Read the model definition and answer for the solid it produces. Units are mm, in the model's axes. A direction names the side the tool comes from. Give positions to 0.01 mm unless a question says otherwise; leave off trailing zeros. Order: outer loops, then holes, each group sorted by start corner. A loop starts at its lowest first (then second) coordinate and runs counter-clockwise, first axis right, second up. Notation, with made-up numbers: M -7.75,29 L 13.25,29 A10 ccw 13.25,43 Z; hole C 72,33.25 d6. An arc over 180 degrees is marked long. One line per item, written item: value. Start each with the question number.
from build123d import *

# Parameters (mm, degrees)
SKETCH1_R           = 1
BOSS_EXTRUDE1_DEPTH = 1.5
FILLET1_R           = 1
FILLET2_R           = 1
FILLET3_R           = 1


with BuildPart() as part:
    # Sketch1 → Boss-Extrude1 (new body)
    with BuildSketch(Plane.XY):
        with BuildLine():
            Line((13.648087548, 15.547724074), (13.648087548, 16.047724074))
            Line((13.648087548, 16.047724074), (-11.216055041, 18.650494389))
            ThreePointArc((-11.216055041, 18.650494389), (-12.440799912, 18.231633219), (-13.152546714, 17.150494389))
            Line((-13.152546714, 17.150494389), (-15.098105849, 17.150494389))
            Line((-15.098105849, 17.150494389), (-15.098105849, 16.150494389))
            Line((-15.098105849, 16.150494389), (-13.152546714, 16.150494389))
            ThreePointArc((-13.152546714, 16.150494389), (-11.545884817, 14.677878786), (-9.547553428, 15.547724074))
            Line((-9.547553428, 15.547724074), (13.648087548, 15.547724074))
        make_face()
        with Locations((-11.216055041, 16.650494389)):
            Circle(SKETCH1_R, mode=Mode.SUBTRACT)
    extrude(amount=BOSS_EXTRUDE1_DEPTH)

    # Fillet1
    fillet1_edges = [part.edges().sort_by_distance(p)[0] for p in [
        (-13.152546714, 16.150494389, 0.75),
    ]]
    fillet(fillet1_edges, radius=FILLET1_R)

    # Fillet2
    fillet2_edges = [part.edges().sort_by_distance(p)[0] for p in [
        (-13.152546714, 17.150494389, 0.75),
    ]]
    fillet(fillet2_edges, radius=FILLET2_R)

    # Fillet3
    fillet3_edges = [part.edges().sort_by_distance(p)[0] for p in [
        (-9.547553428, 15.547724074, 0.75),
    ]]
    fillet(fillet3_edges, radius=FILLET3_R)


solid = part.part
Q1. Find section C-C, the plane y = 18.35. Give the vertices of the cut face in (x, z), then the cut area to 3 significant figures.
Q2. Each of these flat-tipped pins is pushed along its axis until it touches: pin 1 (0.6 mm diameter, centred on x = -14.5, z = 0.5, fed in from +Y); pin 2 (0.8 mm diameter, centred on x = -2, z = 0.5, fed in from -Y). Where does it stop, or does it pass through?
Q3. Consider probe 1 along Y at (x, z) = (-10.75, 0.7); probe 2 along Y at (x, z) = (3.75, 0.7); probe 3 along Y at (x, z) = (-1, 0.3). Determine where each line is inside the solid, lowest interval first.
Q4. Determine the mould class of faces 1 (the cylindrical face through (-13.32, 17.28, 0.76)), 2 (the cylindrical face through (-11.49, 14.67, 0.74)), 3 (the cylindrical face through (-11.35, 17.64, 0.74)) for opening direction Y: released by +Y, released by -Y, zero draft, split by the parting line, or undercut.
Q5. A tool of negligible diameter and unlimited length cuts with its end or side. For faces 4 (the flat face through (-4, 17, 0)), 5 (the flat face through (2, 15.548, 1)), 6 (the flat face through (-14, 17.15, 1)), 7 (the flat face through (-4, 17, 1.5)), 8 (the flat face through (-14, 16.15, 1)), from which of +Z, -Z, +X, -X, +Y, -Y can it reach the whole face along a straight path? Write none if from no direction.
Q6. Find section A-A, the plane z = 0.8. Give the vertices of the cut face in (x, y), then the cut area to 3 significant figures.
Q7. Find section B-B, the plane x = 4.75. Give the vertices of the cut face in (y, z), then the cut area to 3 significant figures.
Evaluation:
1. outline: M -12.27,0 L -8.35,0 L -8.35,1.5 L -12.27,1.5 Z
1. area: 5.89 mm2
2. pin 1: y = 17.15
2. pin 2: y = 15.55
3. probe 1: 14.71 to 15.77, 17.54 to 18.6
3. probe 2: 15.55 to 17.08
3. probe 3: 15.55 to 17.58
4. face 1: released by +Y
4. face 2: released by -Y
4. face 3: undercut
5. face 4: -Z, +X, -X, +Y, -Y
5. face 5: +Z, -Z, +X, -Y
5. face 6: +Z, -Z, -X, +Y
5. face 7: +Z, +X, -X, +Y, -Y
5. face 8: +Z, -Z, -X, -Y
6. outline: M -15.1,16.15 L -13.81,16.15 A1 cw -12.95,15.65 A2 ccw -9.79,15.25 A1 cw -9.08,15.55 L 13.65,15.55 L 13.65,16.05 L -11.22,18.65 A2 ccw -12.95,17.65 A1 cw -13.81,17.15 L -15.1,17.15 Z; hole C -11.22,16.65 d2
6. area: 51.1 mm2
7. outline: M 15.55,0 L 16.98,0 L 16.98,1.5 L 15.55,1.5 Z
7. area: 2.15 mm2
